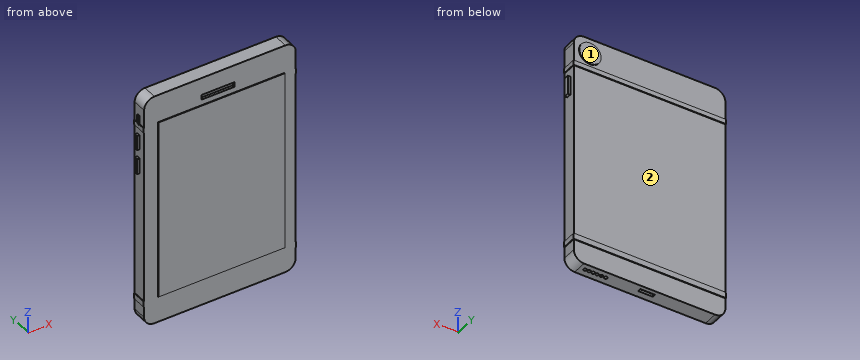
from build123d import *

# Parameters (mm, degrees)
F0_W      = 74.7929699719
F0_H      = 116.6311837733
F1_DEPTH  = 7.112
F2_W      = 2.2798741702
F2_H      = 9.3019269407
F3_DEPTH  = 1.27
F4_W      = 1.6649477184
F4_H      = 7.7697578818
F5_DEPTH  = 1.27
F4_H_2    = 7.214775309
F6_DEPTH  = 1.27
F4_W_2    = 1.2949595693
F4_H_3    = 4.4398605824
F7_DEPTH  = 0.508
F10_W     = 16.2794925272
F10_H     = 2.4049207568
F11_DEPTH = 1.27
F14_R     = 5.08
F15_R     = 5.08
F16_W     = 62.410261482
F16_H     = 89.7654034197
F17_DEPTH = 0.254
F21_R     = 5.3775746227
F22_DEPTH = 0.254
F25_W     = 74.7929699719
F25_H     = 2.4049244821
F26_DEPTH = 0.254
F29_DEPTH = 0.254
F30_DEPTH = 0.254
F31_W     = 74.7929699719
F31_H     = 2.9377117753
F34_DEPTH = 0.254
F32_W     = 7.112
F32_H     = 2.813577652
F35_DEPTH = 0.254
F33_W     = 7.112
F33_H     = 2.8514191508
F36_DEPTH = 0.254
F8_R      = 0.7916480681
F39_DEPTH = 1.27
F9_R      = 0.7862255443
F9_R_2    = 0.7916480681
F9_R_3    = 0.7862255169
F9_R_4    = 0.7902964021
F40_DEPTH = 1.27
F41_W     = 7.3253975715
F41_H     = 1.6351337545
F42_DEPTH = 1.27


# Not quite as in the source:
# - the program builds the solid bodies; features that only make, move or delete a surface that nothing else refers to are left out


with BuildPart() as f1:
    # F0 (on Front) → F1 (new body)
    with BuildSketch(Plane.XZ):
        with Locations((0.7164049894, -7.1640815586)):
            Rectangle(F0_W, F0_H)
    extrude(amount=F1_DEPTH)

    # F2 (on face) → F3 (join)
    with BuildSketch(Plane.YZ.offset(38.1128899753)):
        with Locations((-3.7364399759, 25.567272678)):
            Rectangle(F2_W, F2_H)
    extrude(amount=F3_DEPTH)

    # F4 (on face) → F5 (join)
    with BuildSketch(Plane(origin=(-36.6800799966, 0, 0), x_dir=(0, -1, 0), z_dir=(-1, 0, 0))):
        with Locations((2.8674099594, 15.4470177367)):
            Rectangle(F4_W, F4_H)
    extrude(amount=F5_DEPTH)

    # F4 (on face) → F6 (join)
    with BuildSketch(Plane(origin=(-36.6800799966, 0, 0), x_dir=(0, -1, 0), z_dir=(-1, 0, 0))):
        with Locations((2.8674099594, 27.5641391054)):
            Rectangle(F4_W, F4_H_2)
    extrude(amount=F6_DEPTH)

    # F4 (on face) → F7 (join)
    with BuildSketch(Plane(origin=(-36.6800799966, 0, 0), x_dir=(0, -1, 0), z_dir=(-1, 0, 0))):
        with Locations((3.052404034, 38.941282779)):
            Rectangle(F4_W_2, F4_H_3)
    extrude(amount=F7_DEPTH)

    # F10 (on face) → F11 (cut)
    with BuildSketch(Plane.XZ.offset(7.112)):
        with Locations((-0.1849941909, 41.2537120283)):
            Rectangle(F10_W, F10_H)
    extrude(amount=-F11_DEPTH, mode=Mode.SUBTRACT)

    # F14
    f14_edges = [f1.edges().sort_by_distance(p)[0] for p in [
        (38.11289, -3.556, 51.15151),
    ]]
    fillet(f14_edges, radius=F14_R)

    # F15
    f15_edges = [f1.edges().sort_by_distance(p)[0] for p in [
        (-36.68008, -3.556, 51.15151),
        (-36.68008, -3.556, -65.479673),
        (38.11289, -3.556, -65.479673),
    ]]
    fillet(f15_edges, radius=F15_R)

    # F16 (on face) → F17 (join)
    with BuildSketch(Plane.XZ.offset(7.112)):
        with Locations((1.43471919, -7.7157635242)):
            Rectangle(F16_W, F16_H)
    extrude(amount=F17_DEPTH)

    # F21 (on Front) → F22 (join)
    with BuildSketch(Plane.XZ):
        with Locations((30.1540587097, 43.5661412776)):
            Circle(F21_R)
    extrude(amount=-F22_DEPTH)

    # F25 (on face) → F26 (join)
    with BuildSketch(Plane(origin=(0, 0, 0), x_dir=(-1, 0, 0), z_dir=(0, 1, 0))):
        with Locations((-0.7164049894, 35.7038844377)):
            Rectangle(F25_W, F25_H)
    extrude(amount=F26_DEPTH)

    # F27 (on face) → F29 (join)
    with BuildSketch(Plane.YZ.offset(38.1128899753)):
        Polygon((0.254, 34.5014221966), (0.254, 36.9063466787), (0, 36.9063466787), (-7.112, 36.9063466787), (-7.112, 34.5014221966), (0, 34.5014221966), align=None)
    extrude(amount=F29_DEPTH)

    # F28 (on face) → F30 (join)
    with BuildSketch(Plane(origin=(-36.6800799966, 0, 0), x_dir=(0, -1, 0), z_dir=(-1, 0, 0))):
        Polygon((2.4049242493, 36.9063466787), (0, 36.9063466787), (-0.254, 36.9063466787), (-0.254, 34.5014221966), (0, 34.5014221966), (7.112, 34.5014221966), (7.112, 36.9063466787), (3.6998838186, 36.9063466787), (3.6998838186, 36.7213524878), (2.4049242493, 36.7213524878), align=None)
    extrude(amount=F30_DEPTH)

    # F31 (on face) → F34 (join)
    with BuildSketch(Plane(origin=(0, 0, 0), x_dir=(-1, 0, 0), z_dir=(0, 1, 0))):
        with Locations((-0.7164049894, -53.544729948)):
            Rectangle(F31_W, F31_H)
    extrude(amount=F34_DEPTH)

    # F32 (on face) → F35 (join)
    with BuildSketch(Plane.YZ.offset(38.1128899753)):
        with Locations((-3.556, -53.5610467196)):
            Rectangle(F32_W, F32_H)
    extrude(amount=F35_DEPTH)

    # F33 (on face) → F36 (join)
    with BuildSketch(Plane(origin=(-36.6800799966, 0, 0), x_dir=(0, -1, 0), z_dir=(-1, 0, 0))):
        with Locations((3.556, -53.6269359291)):
            Rectangle(F33_W, F33_H)
    extrude(amount=F36_DEPTH)

    # F8 (on face) → F39 (cut)
    with BuildSketch(Plane(origin=(0, 0, -65.4796734452), x_dir=(1, 0, 0), z_dir=(0, 0, -1))):
        with Locations((20.1854705811, 3.3230686095)):
            Circle(F8_R)
    extrude(amount=-F39_DEPTH, mode=Mode.SUBTRACT)

    # F9 (on face) → F40 (cut)
    with BuildSketch(Plane(origin=(0, 0, -65.4796734452), x_dir=(1, 0, 0), z_dir=(0, 0, -1))):
        with Locations((30.3601529449, 3.3230686095)):
            Circle(F9_R)
        with Locations((28.4177139401, 3.3230686095)):
            Circle(F9_R_2)
        with Locations((26.3827759773, 3.3230686095)):
            Circle(F9_R)
        with Locations((24.4403369725, 3.3230686095)):
            Circle(F9_R_3)
        with Locations((22.3591532558, 3.3230686095)):
            Circle(F9_R_4)
    extrude(amount=-F40_DEPTH, mode=Mode.SUBTRACT)

    # F41 (on face) → F42 (cut)
    with BuildSketch(Plane(origin=(0, 0, -65.4796734452), x_dir=(1, 0, 0), z_dir=(0, 0, -1))):
        with Locations((0.251334277, 2.8914771974)):
            Rectangle(F41_W, F41_H)
    extrude(amount=-F42_DEPTH, mode=Mode.SUBTRACT)


solid = f1.part
Here's how the part is built. I have some questions about the finished solid (model axes, mm). Face numbers are marked on the shaded views. A direction names the side the tool comes from. Round coordinates to 2 decimals unless told otherwise and drop trailing zeros. Write each loop counter-clockwise with the first axis right and the second up, starting at its lowest first coordinate (ties: lowest second). Pieces come first, ordered by that corner, then holes. Notation, with made-up numbers: (27.25, -18.5) -> (75.25, -18.5) arc R17 ccw to (75.25, -4.5) -> close; hole circle Ø2 at (22, -13.75). An arc over 180 degrees is marked (long way). One line per item, written item: value.
1) If I drill on line 1 (X direction, y = -2.25, z = -2); line 2 (Y direction, x = 6, z = -29); line 3 (X direction, y = -2.5, z = 40), over which ranges is the centre line in solid material (lowest first)? Write a range as [from, to].
Filled sheet:
line 1: x = [-36.68, 38.11]
line 2: y = [-7.37, 0]
line 3: x = [-37.19, 38.11]
2) Suppose I cut it at C-C on x = -23.5. List the corners of the cut face in (y, z) for me, plus the area to 3 significant figures.
Filled sheet:
outline: (-7.37, -52.6) -> (-7.11, -52.6) -> (-7.11, -65.48) -> (0, -65.48) -> (0, -55.01) -> (0.25, -55.01) -> (0.25, -52.08) -> (0, -52.08) -> (0, 34.5) -> (0.25, 34.5) -> (0.25, 36.91) -> (0, 36.91) -> (0, 51.15) -> (-7.11, 51.15) -> (-7.11, 37.17) -> (-7.37, 37.17) -> close
area: 854 mm2
3) For the marked faces 1 and 2, which set-ups out of +Z, -Z, +X, -X, +Y, -Y let a thin tool reach every point of the face, with its end or its side?
Filled sheet:
face 1: +Z, -Z, +X, -X, +Y
face 2: +X, -X, +Y
4) Suppose I cut it at B-B on z = -6. List the corners of the cut face in (x, y) for me, plus the area to 3 significant figures.
Filled sheet:
outline: (-36.68, -7.11) -> (-29.77, -7.11) -> (-29.77, -7.37) -> (32.64, -7.37) -> (32.64, -7.11) -> (38.11, -7.11) -> (38.11, 0) -> (-36.68, 0) -> close
area: 548 mm2
5) Suppose I cut it at A-A on x = 6.5. List the corners of the cut face in (y, z) for me.
Filled sheet:
outline: (-7.37, -52.6) -> (-7.11, -52.6) -> (-7.11, -65.48) -> (0, -65.48) -> (0, -55.01) -> (0.25, -55.01) -> (0.25, -52.08) -> (0, -52.08) -> (0, 34.5) -> (0.25, 34.5) -> (0.25, 36.91) -> (0, 36.91) -> (0, 51.15) -> (-7.11, 51.15) -> (-7.11, 42.46) -> (-5.84, 42.46) -> (-5.84, 40.05) -> (-7.11, 40.05) -> (-7.11, 37.17) -> (-7.37, 37.17) -> close
6) Suppose I cut it at D-D on z = 14. List the corners of the cut face in (x, y) for me, plus the area to 3 significant figures.
Filled sheet:
outline: (-37.95, -3.7) -> (-36.68, -3.7) -> (-36.68, -7.11) -> (-29.77, -7.11) -> (-29.77, -7.37) -> (32.64, -7.37) -> (32.64, -7.11) -> (38.11, -7.11) -> (38.11, 0) -> (-36.68, 0) -> (-36.68, -2.03) -> (-37.95, -2.03) -> close
area: 550 mm2
7) I'm going to push flat-ended pins straight in: pin 1 Ø1.4 at (x, z) = (-37.5, 28.5) entering from -Y; pin 2 Ø0.6 at (y, z) = (-6.5, 41.5) entering from -X; pin 3 Ø2 at (y, z) = (-4, -6.5) entering from +X. Where does each tip first touch, or does it pass through?
Filled sheet:
pin 1: stops at y = -3.7
pin 2: stops at x = -36.68
pin 3: stops at x = 38.11
